from build123d import *

# Parameters (mm, degrees)
CYLINDER006_R            = 2.45
CYLINDER006_DEPTH        = 1000
PRISM_DEPTH              = 5
CYLINDER005_R            = 5
CYLINDER005_DEPTH        = 1000
CYLINDER003_R            = 10
CYLINDER003_DEPTH        = 5
CYLINDER004_R            = 7.5
CYLINDER004_DEPTH        = 7
CUBE008_W                = 20
CUBE008_H                = 5
CUBE008_DEPTH            = 13
UNION001_PLACEMENT_ANGLE = 180
CYLINDER001_R            = 10
CYLINDER001_DEPTH        = 5
CYLINDER002_R            = 7.5
CYLINDER002_DEPTH        = 7
CUBE007_W                = 20
CUBE007_H                = 5
CUBE007_DEPTH            = 13
CUBE006_W                = 100
CUBE006_H                = 10
CUBE006_DEPTH            = 100
CUBE005_W                = 100
CUBE005_H                = 10
CUBE005_DEPTH            = 100
CUBE002_W                = 4
CUBE002_H                = 6
CUBE002_DEPTH            = 11
CUBE003_W                = 4
CUBE003_H                = 6
CUBE003_DEPTH            = 11
CUBE004_W                = 4
CUBE004_H                = 6
CUBE004_DEPTH            = 11
CUBE001_W                = 4
CUBE001_H                = 6
CUBE001_DEPTH            = 11
CYLINDER_R               = 3.5
CYLINDER_DEPTH           = 100
CUBE_W                   = 20
CUBE_H                   = 20
CUBE_DEPTH               = 5
CHAMFER_SIZE             = 1.9
CHAMFER001_SIZE          = 1.9
CHAMFER002_SIZE          = 1.9
CHAMFER003_SIZE          = 1.9
FILLET_R                 = 2
FILLET001_R              = 2
FILLET002_R              = 2
FILLET003_R              = 2
FILLET004_R              = 1
FILLET005_R              = 1
FILLET006_R              = 1
FILLET007_R              = 1


with BuildPart() as cylinder006:
    # cylinder006 → cylinder006 (new body)
    with BuildSketch(Plane(origin=(0, 500, -13), x_dir=(1, 0, 0), z_dir=(0, -1, 0))):
        Circle(CYLINDER006_R)
    extrude(amount=CYLINDER006_DEPTH)


with BuildPart() as prism:
    # prism → prism (new body)
    with BuildSketch(Plane(origin=(0, -8.33333, -13), x_dir=(0, 0, -1), z_dir=(0, -1, 0))):
        Polygon((5.79, 0), (2.895, 5.014287), (-2.895, 5.014287), (-5.79, 0), (-2.895, -5.014287), (2.895, -5.014287), align=None)
    extrude(amount=PRISM_DEPTH)


with BuildPart() as union002:
    # cylinder005 → cylinder005 (new body)
    with BuildSketch(Plane.XY.offset(-500)):
        Circle(CYLINDER005_R)
    extrude(amount=CYLINDER005_DEPTH)

    # union002: union cylinder006, prism
    add(cylinder006.part)
    add(prism.part)


with BuildPart() as cylinder003:
    # cylinder003 → cylinder003 (new body)
    with BuildSketch(Plane(origin=(0, 10, -13), x_dir=(1, 0, 0), z_dir=(0, -1, 0))):
        Circle(CYLINDER003_R)
    extrude(amount=CYLINDER003_DEPTH)


with BuildPart() as cylinder004:
    # cylinder004 → cylinder004 (new body)
    with BuildSketch(Plane(origin=(0, 10, -13), x_dir=(1, 0, 0), z_dir=(0, -1, 0))):
        Circle(CYLINDER004_R)
    extrude(amount=CYLINDER004_DEPTH)


with BuildPart() as union001:
    # cube008 → cube008 (new body)
    with BuildSketch(Plane(origin=(-10, -10, -13), x_dir=(1, 0, 0), z_dir=(0, 0, 1))):
        with Locations((10, 2.5)):
            Rectangle(CUBE008_W, CUBE008_H)
    extrude(amount=CUBE008_DEPTH)

    # union001: union cylinder003, cylinder004
    add(cylinder003.part)
    add(cylinder004.part)


with BuildPart() as union001_1:
    # union001 placement: moved
    add(union001.part.rotate(Axis((0, 0, 0), (0, 0, 1)), UNION001_PLACEMENT_ANGLE))


with BuildPart() as cylinder001:
    # cylinder001 → cylinder001 (new body)
    with BuildSketch(Plane(origin=(0, 10, -13), x_dir=(1, 0, 0), z_dir=(0, -1, 0))):
        Circle(CYLINDER001_R)
    extrude(amount=CYLINDER001_DEPTH)


with BuildPart() as cylinder002:
    # cylinder002 → cylinder002 (new body)
    with BuildSketch(Plane(origin=(0, 10, -13), x_dir=(1, 0, 0), z_dir=(0, -1, 0))):
        Circle(CYLINDER002_R)
    extrude(amount=CYLINDER002_DEPTH)


with BuildPart() as difference002:
    # cube007 → cube007 (new body)
    with BuildSketch(Plane(origin=(-10, -10, -13), x_dir=(1, 0, 0), z_dir=(0, 0, 1))):
        with Locations((10, 2.5)):
            Rectangle(CUBE007_W, CUBE007_H)
    extrude(amount=CUBE007_DEPTH)

    # union: union cylinder001, cylinder002
    add(cylinder001.part)
    add(cylinder002.part)

    # Group003: union union001
    add(union001_1.part)

    # difference002: cut union002
    add(union002.part, mode=Mode.SUBTRACT)


with BuildPart() as cube006:
    # cube006 → cube006 (new body)
    with BuildSketch(Plane(origin=(-5.15, 5, -50), x_dir=(-1, 0, 0), z_dir=(0, 0, 1))):
        with Locations((50, 5)):
            Rectangle(CUBE006_W, CUBE006_H)
    extrude(amount=CUBE006_DEPTH)


with BuildPart() as group002:
    # cube005 → cube005 (new body)
    with BuildSketch(Plane(origin=(5.15, -5, -50), x_dir=(1, 0, 0), z_dir=(0, 0, 1))):
        with Locations((50, 5)):
            Rectangle(CUBE005_W, CUBE005_H)
    extrude(amount=CUBE005_DEPTH)

    # Group002: union cube006
    add(cube006.part)


with BuildPart() as cube002:
    # cube002 → cube002 (new body)
    with BuildSketch(Plane(origin=(3, 6, 0), x_dir=(0, 1, 0), z_dir=(0, 0, 1))):
        with Locations((2, 3)):
            Rectangle(CUBE002_W, CUBE002_H)
    extrude(amount=CUBE002_DEPTH)


with BuildPart() as cube003:
    # cube003 → cube003 (new body)
    with BuildSketch(Plane(origin=(-6, 3, 0), x_dir=(-1, 0, 0), z_dir=(0, 0, 1))):
        with Locations((2, 3)):
            Rectangle(CUBE003_W, CUBE003_H)
    extrude(amount=CUBE003_DEPTH)


with BuildPart() as cube004:
    # cube004 → cube004 (new body)
    with BuildSketch(Plane(origin=(-3, -6, 0), x_dir=(0, -1, 0), z_dir=(0, 0, 1))):
        with Locations((2, 3)):
            Rectangle(CUBE004_W, CUBE004_H)
    extrude(amount=CUBE004_DEPTH)


with BuildPart() as group:
    # cube001 → cube001 (new body)
    with BuildSketch(Plane(origin=(6, -3, 0), x_dir=(1, 0, 0), z_dir=(0, 0, 1))):
        with Locations((2, 3)):
            Rectangle(CUBE001_W, CUBE001_H)
    extrude(amount=CUBE001_DEPTH)

    # Group: union cube002, cube003, cube004
    add(cube002.part)
    add(cube003.part)
    add(cube004.part)


with BuildPart() as cylinder:
    # cylinder → cylinder (new body)
    with BuildSketch(Plane.XY.offset(-50)):
        Circle(CYLINDER_R)
    extrude(amount=CYLINDER_DEPTH)


with BuildPart() as fillet007:
    # cube → cube (new body)
    with BuildSketch(Plane(origin=(-10, -10, 0), x_dir=(1, 0, 0), z_dir=(0, 0, 1))):
        with Locations((10, 10)):
            Rectangle(CUBE_W, CUBE_H)
    extrude(amount=CUBE_DEPTH)

    # difference: cut cylinder
    add(cylinder.part, mode=Mode.SUBTRACT)

    # Group001: union Group
    add(group.part)

    # difference001: cut Group002
    add(group002.part, mode=Mode.SUBTRACT)

    # Group004: union difference002
    add(difference002.part)

    # Chamfer
    chamfer_edges = [fillet007.edges().sort_by_distance(p)[0] for p in [
        (6.566963, 3, -9.377156),
    ]]
    chamfer(chamfer_edges, length=CHAMFER_SIZE)

    # Chamfer001
    chamfer001_edges = [fillet007.edges().sort_by_distance(p)[0] for p in [
        (7.5, -3, -13),
    ]]
    chamfer(chamfer001_edges, length=CHAMFER001_SIZE)

    # Chamfer002
    chamfer002_edges = [fillet007.edges().sort_by_distance(p)[0] for p in [
        (-6.566963, -3, -9.377156),
    ]]
    chamfer(chamfer002_edges, length=CHAMFER002_SIZE)

    # Chamfer003
    chamfer003_edges = [fillet007.edges().sort_by_distance(p)[0] for p in [
        (-7.5, 3, -13),
    ]]
    chamfer(chamfer003_edges, length=CHAMFER003_SIZE)

    # Fillet
    fillet_edges = [fillet007.edges().sort_by_distance(p)[0] for p in [
        (-5.15, 5, 2.5),
    ]]
    fillet(fillet_edges, radius=FILLET_R)

    # Fillet001
    fillet001_edges = [fillet007.edges().sort_by_distance(p)[0] for p in [
        (-5.15, -5, 2.5),
    ]]
    fillet(fillet001_edges, radius=FILLET001_R)

    # Fillet002
    fillet002_edges = [fillet007.edges().sort_by_distance(p)[0] for p in [
        (5.15, 5, 2.5),
    ]]
    fillet(fillet002_edges, radius=FILLET002_R)

    # Fillet003
    fillet003_edges = [fillet007.edges().sort_by_distance(p)[0] for p in [
        (5.15, -5, 2.5),
    ]]
    fillet(fillet003_edges, radius=FILLET003_R)

    # Fillet004
    fillet004_edges = [fillet007.edges().sort_by_distance(p)[0] for p in [
        (-10, 10, -4),
    ]]
    fillet(fillet004_edges, radius=FILLET004_R)

    # Fillet005
    fillet005_edges = [fillet007.edges().sort_by_distance(p)[0] for p in [
        (-10, -10, -4),
    ]]
    fillet(fillet005_edges, radius=FILLET005_R)

    # Fillet006
    fillet006_edges = [fillet007.edges().sort_by_distance(p)[0] for p in [
        (-10, -5, -4),
    ]]
    fillet(fillet006_edges, radius=FILLET006_R)

    # Fillet007
    fillet007_edges = [fillet007.edges().sort_by_distance(p)[0] for p in [
        (-10, 5, -4),
    ]]
    fillet(fillet007_edges, radius=FILLET007_R)


solid = fillet007.part
For this review, take the finished solid that the model builds, in its own axes (mm). A direction names the side the tool comes from. Round coordinates to 2 decimals unless told otherwise and drop trailing zeros. Loops run counter-clockwise (first coordinate to the right, second up) from the corner with the lowest first, then second, coordinate; pieces in that order, holes last. Notation, with made-up numbers: (33.5, 6) - (75.5, 6) arc R14 ccw to (75.5, 33) - close; hole circle Ø3 at (-7, 61). An arc over 180 degrees is marked (long way). One line per item, written item: value. Start each with the question number.
Item 1: Take a section at C-C (x = -1.5). State how many separate pieces and enclosed holes the cut face has, plus the area to 3 significant figures.
Item 2: The part is to be moulded in two halves that separate along X. For faces 6 (the flat face through (5, -3, -13)), 7 (the cylindrical face through (0, 8, -23)), 8 (the flat face through (2.542, -9.155, -8.678)), say which applies: +X half, -X half, draft (parallel to the pull), parting line (faces both ways), or undercut.
Item 3: For L1, parallel to X at y = -6.25, z = -13; L2, parallel to Y at x = 7.25, z = 0.5; L3, parallel to Z at x = -2.25, y = 7.75, list the stretches that pass through material, from the lowest coordinate up.
Item 4: For faces 1 (the flat face through (-5, -3, -13)), 2 (the cylindrical face through (9.699, -5.285, -4.126)), 3 (the cylindrical face through (5.72, 4.4, 2.54)), 4 (the flat face through (4, 5, -6)), 5 (the flat face through (1.7, 3.4, 0)), list the 3-axis set-ups (+Z, -Z, +X, -X, +Y, -Y) from which the entire face can be reached by the end or side of a thin tool; tool diameter is ignored.
Item 5: Take a section at B-B (y = 0). Give the boundary of the cut face in (x, z), plus the area to 3 significant figures.
Item 6: Clearance check with flat-ended pins moving along their axes: pin 1 Ø1.5 at (y, z) = (1.5, 3) entering from +X; pin 2 Ø3 at (x, z) = (1, -13) entering from -Y; pin 3 Ø2 at (y, z) = (-7, 7) entering from -X. State where each tip first meets the part, or that it passes through.
Item 7: Take a section at A-A (z = 9.5). Give the boundary of the cut face in (x, y), plus the area to 3 significant figures.
Answer below:
1. separate pieces: 4
1. enclosed holes: 0
1. area: 301 mm2
2. face 6: draft
2. face 7: parting line
2. face 8: undercut
3. L1: x = -10 to -2.45, 2.45 to 10
3. L2: y = -10 to -5, 5 to 10
3. L3: z = -22.74 to -13.97, -12.03 to 11
4. face 1: -Z, +X, -X
4. face 2: +Z, -Z, +X
4. face 3: +Z, +X
4. face 4: none
4. face 5: +X, -X
5. outline: (-5.15, 0) - (-3.5, 0) - (-3.5, 5) - (-5.15, 5) - close; (3.5, 0) - (5.15, 0) - (5.15, 5) - (3.5, 5) - close
5. area: 16.5 mm2
6. pin 1: stops at x = 5.15
6. pin 2: stops at y = -8.33
6. pin 3: stops at x = -3
7. outline: (-3, -10) - (3, -10) - (3, -6) - (-3, -6) - close; (-3, 6) - (3, 6) - (3, 10) - (-3, 10) - close
7. area: 48.0 mm2
